The figure shows three views and two pictorial views of one solid part (mm, origin at its lowest corner). Answer the questions. A direction names the side the tool comes from. Coordinates: 2 decimals unless noted, no trailing zeros. Order: outer loops, then holes, each group sorted by start corner. A loop starts at its lowest first (then second) coordinate and runs counter-clockwise, first axis right, second up.
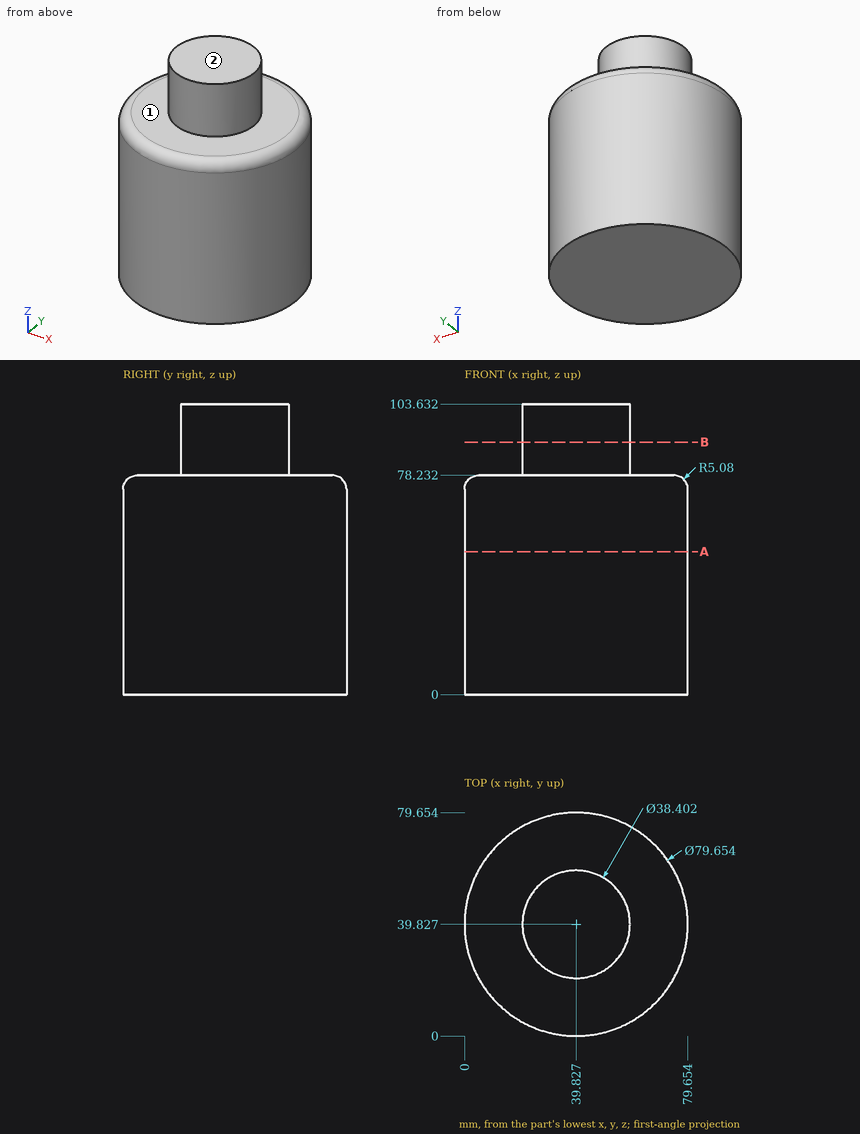
Q1. The part is cut by section B-B, the plane z = 90. Determine the outline of the cut face in (x, y), then the cut area to 3 significant figures.
Q2. Straight lines are drawn through the part: L1, parallel to Z at x = 12, y = 36; L2, parallel to Y at x = 17, z = 63 (1 decimal); L3, parallel to X at y = 26.5, z = 54.5 (1 decimal). For each, find the intervals that lie inside material, in ascending order.
Q3. Which of the six approach directions +Z, -Z, +X, -X, +Y, -Y give full straight-line access (tool end or side, diameter ignored) to the marked faces 1 and 2?
Q4. Each of these flat-tipped pins is pushed along its axis until it touches: P1, Ø5, axis at x = 48, y = 11.5, coming from the +Z side; P2, Ø6, axis at y = 13, z = 42.5, coming from the +X side; P3, Ø3, axis at y = 65, z = 48, coming from the -X side; P4, Ø2, axis at x = 49.5, y = 19.5, coming from the -Z side. Where does it stop, or does it pass through?
Q5. The part is cut by section A-A, the plane z = 51. Determine the outline of the cut face in (x, y) (1 decimal).
Computed values:
1. outline: circle Ø38.4 at (39.83, 39.83)
1. area: 1,160 mm2
2. L1: z = 0 to 78.23
2. L2: y = 7.2 to 72.5
2. L3: x = 2.3 to 77.4
3. face 1: +Z
3. face 2: +Z, +X, -X, +Y, -Y
4. P1: stops at z = 78.23
4. P2: stops at x = 71.74
4. P3: stops at x = 7.8
4. P4: stops at z = 0
5. outline: circle Ø79.7 at (39.8, 39.8)
